from build123d import *
from OCP.BRepFilletAPI import BRepFilletAPI_MakeChamfer

# Parameters (mm, degrees)
EXTRUDE_1_DEPTH        = 40
SKETCH_2_R             = 6.5
CUT_EXTRUDE_1_DEPTH    = 80
CHAMFER_1_SIZE         = 3
CHAMFER_1_SIZE2        = 2.154045129
HOLE_WIZARD_M8_1_D     = 6.8
HOLE_WIZARD_M8_1_DEPTH = 17.707073895
HOLE_WIZARD_M8_1_TIP   = 2.042926105


with BuildPart() as part:
    # 草图1 → 凸台-拉伸1 (new, symmetric)
    with BuildSketch(Plane.XY):
        Polygon((0, 0), (-43, 0), (-45, 2), (-128.585786438, 2), (-130, 0.585786438), (-131.414213562, 2), (-130, 3.414213562), (-130, 37), (-160, 37), (-160, -18), (-27.5, -18), (-27.5, -14.414213562), (-28.914213562, -13), (-27.5, -11.585786438), (-26.085786438, -13), (26.085786438, -13), (27.5, -11.585786438), (28.914213562, -13), (27.5, -14.414213562), (27.5, -18), (160, -18), (160, 37), (105.068765597, 37), (128.585786438, 3.414213562), (130, 2), (128.585786438, 0.585786438), (127.171572875, 2), (70, 2), (68, 0), align=None)
    extrude(amount=EXTRUDE_1_DEPTH, both=True)

    # 草图2 → 切除-拉伸1 (cut)
    with BuildSketch(Plane(origin=(0, 2, 0), x_dir=(1, 0, 0), z_dir=(0, 1, 0))):
        with Locations(Location((-119, 25, 0), (0, 0, 180))):
            Circle(SKETCH_2_R)
        with Locations(Location((-119, -25, 0), (0, 0, 180))):
            Circle(SKETCH_2_R)
    extrude(amount=-CUT_EXTRUDE_1_DEPTH, mode=Mode.SUBTRACT)

    # 倒角1: one chamfer whose edges measure the first distance from different faces: ONE call of the kernel's chamfer builder (chamfer() names one face for all edges)
    chamfer_1_edges_1 = [part.edges().sort_by_distance(p)[0] for p in [
        (105.068765597, 37, 0),
    ]]
    chamfer_1_side_1 = [part.faces().sort_by_distance(p)[0] for p in [
        (132.534382799, 37, 0),
    ]]
    chamfer_1_edges_2 = [part.edges().sort_by_distance(p)[0] for p in [
        (160, 37, 0),
        (160, -18, 0),
        (-160, -18, 0),
        (-160, 37, 0),
        (-130, 37, 0),
    ]]
    chamfer_1 = BRepFilletAPI_MakeChamfer(part.part.solid().wrapped)
    for e in chamfer_1_edges_1:
        chamfer_1.Add(CHAMFER_1_SIZE, CHAMFER_1_SIZE2, e.wrapped, chamfer_1_side_1[0].wrapped)  # the first distance lies on this face
    for e in chamfer_1_edges_2:
        chamfer_1.Add(CHAMFER_1_SIZE, e.wrapped)
    add(Compound.cast(chamfer_1.Shape()), mode=Mode.REPLACE)

    # M8 螺纹孔1
    with Locations(Plane(origin=(-17.5, 0, -27.5), x_dir=(1, 0, 0), z_dir=(0, 1, 0))):
        with Locations((0, 0), (35, 0), (35, -55), (0, -55)):
            Hole(HOLE_WIZARD_M8_1_D / 2, depth=HOLE_WIZARD_M8_1_DEPTH)
            with Locations((0, 0, -(HOLE_WIZARD_M8_1_DEPTH + HOLE_WIZARD_M8_1_TIP / 2))):  # 118° drill point
                Cone(0, HOLE_WIZARD_M8_1_D / 2, HOLE_WIZARD_M8_1_TIP, mode=Mode.SUBTRACT)


solid = part.part
The model under review builds one solid part; all positions refer to its coordinate system, in mm. A direction names the side the tool comes from. Coordinates: 2 decimals unless noted, no trailing zeros. Order: outer loops, then holes, each group sorted by start corner. A loop starts at its lowest first (then second) coordinate and runs counter-clockwise, first axis right, second up. Notation, with made-up numbers: (2, 81.5) -> (28, 81.5) arc R17 cw to (28, 85.5) -> close; hole circle Ø10 at (50.5, 69). An arc over 180 degrees is marked (long way). Answer in a Markdown table with one row per item.
(1) Insertion check: pin 1 (17 mm diameter, centred on x = 102.5, z = 15, fed in from +Y); pin 2 (9 mm diameter, centred on x = -17.5, z = 27.5, fed in from +Y); pin 3 (9 mm diameter, centred on x = 17.5, z = 27.5, fed in from -Y); pin 4 (10.5 mm diameter, centred on x = -119, z = 25, fed in from +Y). Each pin has a flat end and moves straight along its axis. Give the tip position at first contact, or say it passes through.
Answers:
| item | result |
|---|---|
| pin 1 | y = 37 |
| pin 2 | y = 0 |
| pin 3 | y = -13 |
| pin 4 | through |
(2) The part is to be moulded in two halves that separate along Y. For faces 4 (the flat face through (117.289, 19.548, 0.56)), 5 (the cylindrical face through (-112.506, -7.86, -24.714)), 6 (the flat face through (-93, -18, 1)), 7 (the flat face through (13, 0, 1)), say which applies: +Y half, -Y half, draft (parallel to the pull), parting line (faces both ways), or undercut.
Answers:
| item | result |
|---|---|
| face 4 | undercut |
| face 5 | draft |
| face 6 | -Y half |
| face 7 | +Y half |
(3) Wall thickness on line 1 along Z through (x, y) = (-115, 1); line 2 along Z through (x, y) = (17, -3); line 3 along X through (y, z) = (-5, 27): over which ranges is each line inside the solid? List them lowest first.
Answers:
| item | result |
|---|---|
| line 1 | -40 to -30.12, -19.88 to 19.88, 30.12 to 40 |
| line 2 | -40 to -30.86, -24.14 to 24.14, 30.86 to 40 |
| line 3 | -160 to -125.18, -112.82 to -20.86, -14.14 to 14.14, 20.86 to 160 |
(4) Consider section D-D (y = 11). Write out the cut boundary in (x, z).
Answers:
| item | result |
|---|---|
| outline | (-160, -40) -> (-130, -40) -> (-130, 40) -> (-160, 40) -> close; (123.27, -40) -> (160, -40) -> (160, 40) -> (123.27, 40) -> close |
(5) Consider section B-B (y = -7.5). Write out the cut boundary in (x, z), plus the area to 3 significant figures.
Answers:
| item | result |
|---|---|
| outline | (-160, -40) -> (160, -40) -> (160, 40) -> (-160, 40) -> close; hole circle Ø13 at (-119, -25); hole circle Ø13 at (-119, 25); hole circle Ø6.8 at (-17.5, -27.5); hole circle Ø6.8 at (-17.5, 27.5); hole circle Ø6.8 at (17.5, -27.5); hole circle Ø6.8 at (17.5, 27.5) |
| area | 25,200 mm² |
(6) Consider section A-A (x = -119). Write out the cut boundary in (y, z).
Answers:
| item | result |
|---|---|
| outline | (-18, -40) -> (2, -40) -> (2, -31.5) -> (-18, -31.5) -> close; (-18, -18.5) -> (2, -18.5) -> (2, 18.5) -> (-18, 18.5) -> close; (-18, 31.5) -> (2, 31.5) -> (2, 40) -> (-18, 40) -> close |
(7) Machinability: for faces 1 (the flat face through (0, -13, 1)), 2 (the flat face through (-86, 2, 1)), 3 (the flat face through (99, 2, 1)), which of the approach directions +Z, -Z, +X, -X, +Y, -Y give a long, thin tool a straight path to every point of the face, cutting with its end or side? Answer none if there is none.
Answers:
| item | result |
|---|---|
| face 1 | +Z, -Z, -Y |
| face 2 | +Z, -Z, +Y |
| face 3 | +Z, -Z |
